Source: CAD feature listing. Evaluate the final solid. Frame: model axes, mm. A direction names the side the tool comes from. Round coordinates to 2 decimals unless told otherwise and drop trailing zeros. Write each loop counter-clockwise with the first axis right and the second up, starting at its lowest first coordinate (ties: lowest second). Pieces come first, ordered by that corner, then holes. Notation, with made-up numbers: M 60.5,-7 L 73.5,-7 A21 cw 73.5,1 Z; hole C 62.5,-21 d2. An arc over 180 degrees is marked long. Answer in a Markdown table with one row per item.
from build123d import *

# Parameters (mm, degrees)
CYLINDER1760_R               = 9
CYLINDER1760_DEPTH           = 4
CYLINDER1760_PLACEMENT_ANGLE = 225
BOX711_W                     = 28.8
BOX711_H                     = 2
BOX711_DEPTH                 = 4
COMPOUND890_PLACEMENT_ANGLE  = 225
CYLINDER1692_R               = 1.5
CYLINDER1692_DEPTH           = 60
CYLINDER1689_R               = 1.5
CYLINDER1689_DEPTH           = 60
CYLINDER1690_R               = 1.5
CYLINDER1690_DEPTH           = 60
CYLINDER1691_R               = 1.5
CYLINDER1691_DEPTH           = 60
COMPOUND833_PLACEMENT_ANGLE  = 225
CYLINDER2367_R               = 4
CYLINDER2367_DEPTH           = 4
CYLINDER2367_PLACEMENT_ANGLE = 225
BOX930_W                     = 42
BOX930_H                     = 24
BOX930_DEPTH                 = 2
COMPOUND818_PLACEMENT_ANGLE  = 225
CHAMFER058_SIZE              = 2
CHAMFER058_ROLL_ANGLE        = 180
CHAMFER058_PLACEMENT_ANGLE   = -135.000066


with BuildPart() as obj1:
    # Cylinder1760 → Cylinder1760 (new body)
    with BuildSketch(Plane.XY):
        Circle(CYLINDER1760_R)
    extrude(amount=CYLINDER1760_DEPTH)


with BuildPart() as obj1_1:
    # Cylinder1760 placement: moved
    add(obj1.part.moved(Location((63.64, -63.64, 64))).rotate(Axis((63.64, -63.64, 64), (0, 0, 1)), CYLINDER1760_PLACEMENT_ANGLE))


with BuildPart() as compound890:
    # Box711 → Box711 (new body)
    with BuildSketch(Plane(origin=(-14.4, 10, 24), x_dir=(1, 0, 0), z_dir=(0, 0, 1))):
        with Locations((14.4, 1)):
            Rectangle(BOX711_W, BOX711_H)
    extrude(amount=BOX711_DEPTH)


with BuildPart() as compound890_1:
    # Compound890 placement: moved
    add(compound890.part.moved(Location((63.64, -63.64, 38))).rotate(Axis((63.64, -63.64, 38), (0, 0, 1)), COMPOUND890_PLACEMENT_ANGLE))


with BuildPart() as obj2:
    # Cylinder1692 → Cylinder1692 (new body)
    with BuildSketch(Plane(origin=(18, 85, -57), x_dir=(1, 0, 0), z_dir=(0, 0, 1))):
        Circle(CYLINDER1692_R)
    extrude(amount=CYLINDER1692_DEPTH)


with BuildPart() as obj3:
    # Cylinder1689 → Cylinder1689 (new body)
    with BuildSketch(Plane(origin=(-18, 85, -57), x_dir=(1, 0, 0), z_dir=(0, 0, 1))):
        Circle(CYLINDER1689_R)
    extrude(amount=CYLINDER1689_DEPTH)


with BuildPart() as obj4:
    # Cylinder1690 → Cylinder1690 (new body)
    with BuildSketch(Plane(origin=(-18, 95, -57), x_dir=(1, 0, 0), z_dir=(0, 0, 1))):
        Circle(CYLINDER1690_R)
    extrude(amount=CYLINDER1690_DEPTH)


with BuildPart() as compound833:
    # Cylinder1691 → Cylinder1691 (new body)
    with BuildSketch(Plane(origin=(18, 95, -57), x_dir=(1, 0, 0), z_dir=(0, 0, 1))):
        Circle(CYLINDER1691_R)
    extrude(amount=CYLINDER1691_DEPTH)

    # Compound833: union obj2, obj3, obj4
    add(obj2.part)
    add(obj3.part)
    add(obj4.part)


with BuildPart() as compound833_1:
    # Compound833 placement: moved
    add(compound833.part.moved(Location((0, 0, 100))).rotate(Axis((0, 0, 100), (0, 0, 1)), COMPOUND833_PLACEMENT_ANGLE))


with BuildPart() as obj5:
    # Cylinder2367 → Cylinder2367 (new body)
    with BuildSketch(Plane.XY):
        Circle(CYLINDER2367_R)
    extrude(amount=CYLINDER2367_DEPTH)


with BuildPart() as obj5_1:
    # Cylinder2367 placement: moved
    add(obj5.part.moved(Location((63.64, -63.64, 76))).rotate(Axis((63.64, -63.64, 76), (0, 0, 1)), CYLINDER2367_PLACEMENT_ANGLE))


with BuildPart() as g_mini_encoder_washer:
    # Box930 → Box930 (new body)
    with BuildSketch(Plane(origin=(-21, -12, 34), x_dir=(1, 0, 0), z_dir=(0, 0, 1))):
        with Locations((21, 12)):
            Rectangle(BOX930_W, BOX930_H)
    extrude(amount=BOX930_DEPTH)


with BuildPart() as g_mini_encoder_washer_1:
    # Compound818 placement: moved
    add(g_mini_encoder_washer.part.moved(Location((63.64, -63.64, 42))).rotate(Axis((63.64, -63.64, 42), (0, 0, 1)), COMPOUND818_PLACEMENT_ANGLE))

    # Cut472: cut obj5
    add(obj5_1.part, mode=Mode.SUBTRACT)


with BuildPart() as g_mini_encoder_washer_2:
    # Cut472 placement: moved
    add(g_mini_encoder_washer_1.part.moved(Location((0, 0, -10))))

    # Cut481: cut Compound833
    add(compound833_1.part, mode=Mode.SUBTRACT)


with BuildPart() as g_mini_encoder_washer_3:
    # Cut481 placement: moved
    add(g_mini_encoder_washer_2.part.moved(Location((0, 0, -3))))

    # Cut522: cut Compound890
    add(compound890_1.part, mode=Mode.SUBTRACT)

    # Cut523: cut obj1
    add(obj1_1.part, mode=Mode.SUBTRACT)

    # Chamfer058
    chamfer058_edges = [g_mini_encoder_washer_3.edges().sort_by_distance(p)[0] for p in [
        (86.974524, -57.276039, 64),
        (57.276039, -86.974524, 64),
    ]]
    chamfer(chamfer058_edges, length=CHAMFER058_SIZE)


with BuildPart() as g_mini_encoder_washer_4:
    # Chamfer058 roll: moved
    add(g_mini_encoder_washer_3.part.rotate(Axis((0, 0, 0), (1, 0, 0)), CHAMFER058_ROLL_ANGLE))


with BuildPart() as g_mini_encoder_washer_5:
    # Chamfer058 placement: moved
    add(g_mini_encoder_washer_4.part.moved(Location((0, 6, 48))).rotate(Axis((0, 6, 48), (0, 0, 1)), CHAMFER058_PLACEMENT_ANGLE))


solid = g_mini_encoder_washer_5.part
Q1. Section D-D (y = -91.75). Return loops of the section in (x, z).
Solutions:
| item | result |
|---|---|
| outline | M -21,-17 L -4.58,-17 L -4.58,-16 L 4.58,-16 L 4.58,-17 L 21,-17 L 21,-15 L -21,-15 Z |
Q2. Section A-A (y = -81). Return loops of the section in (x, z).
Solutions:
| item | result |
|---|---|
| outline | M -21,-17 L -8.49,-17 L -8.49,-16 L -2.65,-16 L -2.65,-15 L -21,-15 Z; M 2.65,-16 L 8.48,-16 L 8.48,-17 L 21,-17 L 21,-15 L 2.65,-15 Z |
Q3. Pull-direction query (Y, two-part tool) for faces 3 (the cylindrical face through (-18.195, -80.487, -15.986)), 4 (the flat face through (-20, -95, -16)), 5 (the flat face through (-5, -76, -17)), 6 (the cylindrical face through (4.84, -91.59, -16.49)); classes: pulls with the +Y half, pulls with the -Y half, needs draft (parallel to the pull), parting line crosses it, or undercut.
Solutions:
| item | result |
|---|---|
| face 3 | undercut |
| face 4 | pulls with the -Y half |
| face 5 | needs draft |
| face 6 | undercut |
Q4. Material intervals for probe 1 along Y at (x, z) = (-18, -16.75); probe 2 along X at (y, z) = (-89.5, -15.35); probe 3 along X at (y, z) = (-78.75, -15.05), sorted ascending.
Solutions:
| item | result |
|---|---|
| probe 1 | y = -96 to -90.5, -87.5 to -80.5, -77.5 to -72 |
| probe 2 | x = -21 to -19.41, -16.59 to 16.59, 19.41 to 21 |
| probe 3 | x = -21 to -19.48, -16.52 to 16.52, 19.48 to 21 |
Q5. Section C-C (z = -15.4). Return loops of the section in (x, y), and give its area (3 significant figures).
Solutions:
| item | result |
|---|---|
| outline | M -21,-94 L -19,-96 L -14.4,-96 L -14.4,-94 L 14.4,-94 L 14.4,-96 L 19,-96 L 21,-94 L 21,-72 L -21,-72 Z; hole C -18,-89 d3; hole C -18,-79 d3; hole C 0,-84 d8; hole C 18,-89 d3; hole C 18,-79 d3 |
| area | 868 mm2 |
Q6. Contact query for flat-ended pins moving along their axis: pin 1 Ø0.6 at (x, z) = (6, -16) entering from -Y; pin 2 Ø2.5 at (x, y) = (-18, -89) entering from -Z. Output: stop coordinate, or through.
Solutions:
| item | result |
|---|---|
| pin 1 | stops at y = -94 |
| pin 2 | passes through |
Q7. Section B-B (x = -2). Return loops of the section in (y, z).
Solutions:
| item | result |
|---|---|
| outline | M -94,-17 L -92.78,-17 L -92.78,-16 L -87.46,-16 L -87.46,-15 L -94,-15 Z; M -80.54,-16 L -75.23,-16 L -75.23,-17 L -72,-17 L -72,-15 L -80.54,-15 Z |
Q8. Access query for faces 1 (the cylindrical face through (18.69, -87.67, -15.99)), 2 (the flat face through (4, -82, -16)). Directions: +Z, -Z, +X, -X, +Y, -Y. A direction counts if a zero-diameter tool reaches every point of the face in a straight line with its end or side. Return the directions, or none.
Solutions:
| item | result |
|---|---|
| face 1 | +Z, -Z |
| face 2 | -Z |
